The model under review builds one solid part; all positions refer to its coordinate system, in mm. Face numbers are marked on the shaded views. A direction names the side the tool comes from. Round coordinates to 2 decimals unless told otherwise and drop trailing zeros. Order: outer loops, then holes, each group sorted by start corner. A loop starts at its lowest first (then second) coordinate and runs counter-clockwise, first axis right, second up. Notation, with made-up numbers: (76.25, 65) -> (125.25, 65) arc R27 ccw to (125.25, 92) -> close; hole circle Ø11 at (82, 24.5). An arc over 180 degrees is marked (long way). Put each result on its own line as item: value. Start each with the question number.
from build123d import *

# Parameters (mm, degrees)
SKETCH_1_R          = 3.25
SKETCH_1_R_2        = 1.5
EXTRUDE_1_DEPTH     = 12.5
SKETCH_2_R          = 12.5
CUT_EXTRUDE_1_DEPTH = 2
CUT_EXTRUDE_START   = -6.5
SKETCH_3_R          = 12.5
CUT_EXTRUDE_2_DEPTH = 6.5
EXTRUDE_2_REACH     = 40.836
FILLET_1_R          = 1
FILLET_2_R          = 3


with BuildPart() as part:
    # 草图1 → 凸台-拉伸1 (new body)
    with BuildSketch(Plane(origin=(0, 0, 0), x_dir=(0, 0, -1), z_dir=(1, 0, 0))):
        with BuildLine():
            Line((2.190082511, 13.827636768), (25.525125149, 10.1317291))
            Line((25.525125149, 10.1317291), (32.828427125, 2.828427125))
            ThreePointArc((32.828427125, 2.828427125), (32.828427125, -2.828427125), (27.171572875, -2.828427125))
            Line((27.171572875, -2.828427125), (24.343145751, 0))
            Line((24.343145751, 0), (14, 0))
            ThreePointArc((14, 0), (-10.645683518, -9.092272677), (2.190082511, 13.827636768))
        make_face()
        Circle(SKETCH_1_R, mode=Mode.SUBTRACT)
        with Locations((0, 8)):
            Circle(SKETCH_1_R_2, mode=Mode.SUBTRACT)
        with Locations((8, 0)):
            Circle(SKETCH_1_R_2, mode=Mode.SUBTRACT)
        with Locations((0, -8)):
            Circle(SKETCH_1_R_2, mode=Mode.SUBTRACT)
        with Locations((-8, 0)):
            Circle(SKETCH_1_R_2, mode=Mode.SUBTRACT)
        with Locations((30, 0)):
            Circle(SKETCH_1_R_2, mode=Mode.SUBTRACT)
    extrude(amount=EXTRUDE_1_DEPTH)

    # 草图2 → 切除-拉伸1 (cut)
    with BuildSketch(Plane.ZY):
        Circle(SKETCH_2_R)
    extrude(amount=-CUT_EXTRUDE_1_DEPTH, mode=Mode.SUBTRACT)

    # 草图3 → 切除-拉伸2 (cut)
    with BuildSketch(Plane(origin=(12.5, 0, 0), x_dir=(0, 0, -1), z_dir=(1, 0, 0)).offset(CUT_EXTRUDE_START)):
        with Locations(Location((0, 0, 0), (0, 0, 180))):
            Circle(SKETCH_3_R)
        with BuildLine():
            Line((14, 2), (13.856406461, 2))
            ThreePointArc((13.856406461, 2), (12.232187693, 6.809815287), (8.999535493, 10.724195117))
            Line((8.999535493, 10.724195117), (24.570417428, 8.258009697))
            Line((24.570417428, 8.258009697), (28.96472382, 3.863703305))
            ThreePointArc((28.96472382, 3.863703305), (27.171572875, 2.828427125), (26.136296695, 1.03527618))
            Line((26.136296695, 1.03527618), (25.171572875, 2))
            Line((25.171572875, 2), (14, 2))
        make_face()
    extrude(amount=CUT_EXTRUDE_2_DEPTH, mode=Mode.SUBTRACT)

    # 草图4 → 凸台-拉伸2 (add, up to next)
    with BuildSketch(Plane(origin=(12.5, 0, 0), x_dir=(0, 0, -1), z_dir=(1, 0, 0)), mode=Mode.PRIVATE) as extrude_2_sk1:
        Polygon((25.171572875, 2), (17.848994346, 9.32257853), (14.488282804, 9.854862946), (22.343145751, 2), align=None)
    extrude_2_tool1 = extrude(extrude_2_sk1.sketch, amount=-EXTRUDE_2_REACH, mode=Mode.PRIVATE) - part.part
    add(extrude_2_tool1.solids().sort_by_distance((12.5, 5.795916, -19.944911))[0])

    # 圆角1
    fillet_1_edges = [part.edges().sort_by_distance(p)[0] for p in [
        (9.25, 2, -22.343145751),
        (9.25, 9.854862946, -14.488282804),
        (9.25, 9.32257853, -17.848994346),
        (9.25, 2, -13.856406461),
        (9.25, 10.724195117, -8.999535493),
        (9.25, 8.258009697, -24.570417428),
        (9.25, 3.863703305, -28.96472382),
        (9.25, 1.03527618, -26.136296695),
    ]]
    fillet(fillet_1_edges, radius=FILLET_1_R)

    # 圆角2
    fillet_2_edges = [part.edges().sort_by_distance(p)[0] for p in [
        (6.25, 10.1317291, -25.525125149),
        (6.25, 0, -24.343145751),
        (6.25, 0, -14),
    ]]
    fillet(fillet_2_edges, radius=FILLET_2_R)


solid = part.part
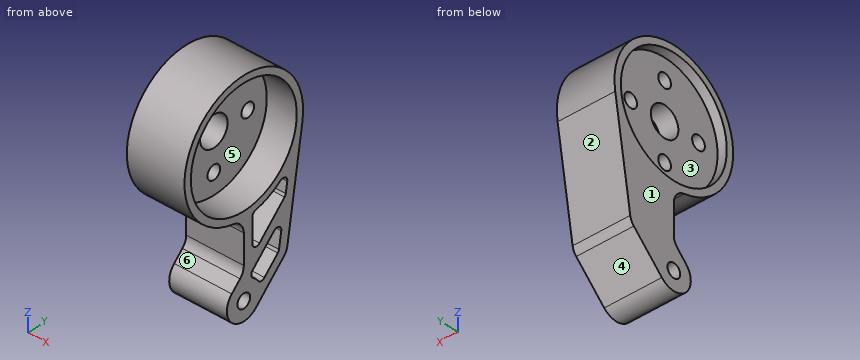
Q1. Take a section at B-B on x = 3.25. Give the boundary of the cut face in (y, z), and give its area (3 significant figures).
Q2. Take a section at A-A on z = 0. Give the boundary of the cut face in (x, y).
Q3. Take a section at C-C on y = -7.5. Give the boundary of the cut face in (x, z).
Q4. For the marked faces 4, 5 and 6, list the 3-axis set-ups (+Z, -Z, +X, -X, +Y, -Y) from which the entire face can be reached by the end or side of a thin tool; tool diameter is ignored.
Q5. Draft analysis for pull direction Z (two halves, no side actions). For the marked faces 1, 2 and 3, state which applies: +Z half, -Z half, draft (parallel to the pull), parting line (faces both ways), or undercut.
Q6. Wall thickness on probe 1 along Y at (x, z) = (3.95, 0); probe 2 along Y at (x, z) = (11, 0); probe 3 along Z at (x, y) = (11.5, 8): over which ranges is each line inside the solid? List them lowest first. Write a range as [from, to].
Q7. Take a section at D-D on z = -30. Give the boundary of the cut face in (x, y), and give its area (3 significant figures).
Q8. Clearance check with flat-ended pins moving along their axes: pin 1 Ø6.5 at (y, z) = (5, -15) entering from +X; pin 2 Ø2 at (x, z) = (6, -13) entering from +Y; pin 3 Ø7.5 at (y, z) = (-5.5, -4) entering from +X; pin 4 Ø6 at (x, z) = (2.5, -12) entering from +Y. State where each tip first meets the part, or that it passes through.
Calculated:
1. outline: (-2.83, -27.17) arc R4 ccw to (2.83, -32.83) -> (9.44, -26.21) arc R3 ccw to (10.28, -24.56) -> (13.83, -2.19) arc R14 ccw (long way) to (-2.47, -13.78) arc R3 cw to (0, -16.73) -> (0, -23.1) arc R3 cw to (-0.88, -25.22) -> close; hole circle Ø3 at (-8, 0); hole circle Ø6.5 at (0, 0); hole circle Ø3 at (0, -30); hole circle Ø3 at (0, -8); hole circle Ø3 at (0, 8); hole circle Ø3 at (8, 0)
1. area: 781 mm²
2. outline: (0, -14) -> (12.5, -14) -> (12.5, -12.5) -> (6, -12.5) -> (6, -9.5) -> (2, -9.5) -> (2, -12.5) -> (0, -12.5) -> close; (0, 12.5) -> (2, 12.5) -> (2, 9.5) -> (6, 9.5) -> (6, 12.5) -> (12.5, 12.5) -> (12.5, 14) -> (0, 14) -> close; (2, -6.5) -> (6, -6.5) -> (6, -3.25) -> (2, -3.25) -> close; (2, 3.25) -> (6, 3.25) -> (6, 6.5) -> (2, 6.5) -> close
3. outline: (0, -11.82) -> (12.5, -11.82) -> (12.5, -10) -> (6, -10) -> (6, -1.41) -> (2, -1.41) -> (2, -10) -> (0, -10) -> close; (0, 10) -> (2, 10) -> (2, 1.41) -> (6, 1.41) -> (6, 10) -> (12.5, 10) -> (12.5, 11.82) -> (0, 11.82) -> close
4. face 4: -Z, +X, -X, +Y
4. face 5: +X
4. face 6: +X, -X, -Y
5. face 1: draft
5. face 2: -Z half
5. face 3: undercut
6. probe 1: y = [-14, -9.5], [-6.5, -3.25], [3.25, 6.5], [9.5, 14]
6. probe 2: y = [-14, -12.5], [12.5, 14]
6. probe 3: z = [-27.66, -24.83], [-19.74, -16.34], [-11.49, -9.6], [9.6, 11.49]
7. outline: (0, -4) -> (12.5, -4) -> (12.5, -1.5) -> (0, -1.5) -> close; (0, 1.5) -> (12.5, 1.5) -> (12.5, 5.66) -> (0, 5.66) -> close
7. area: 83.2 mm²
8. pin 1: stops at x = 12.5
8. pin 2: stops at y = 12.27
8. pin 3: stops at x = 6
8. pin 4: stops at y = 12.75
